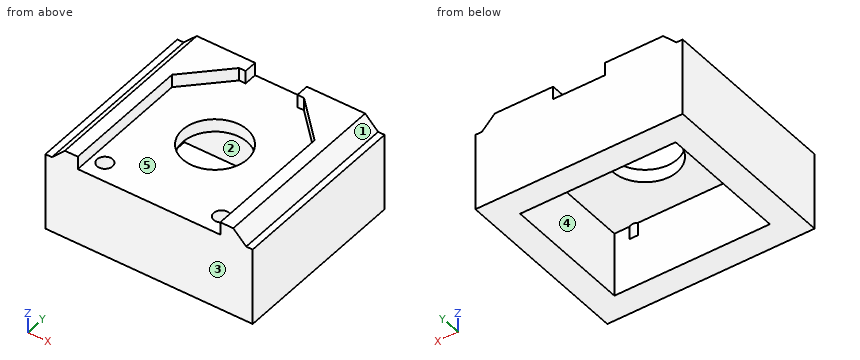
Autodesk Inventor part; units mm, degrees
ref_plane "YZ Plane" through (0, 0, 0) normal (1, 0, 0) x (0, 1, 0)
ref_plane "XZ Plane" through (0, 0, 0) normal (0, 1, 0) x (-1, 0, 0)
ref_plane "XY Plane" through (0, 0, 0) normal (0, 0, 1) x (1, 0, 0)
sketch "Sketch1" plane through (0, 0, 0) normal (0, 0, 1) x (1, 0, 0)
  line L0 (-14.0621, 11.3836) -> (-2.0621, 11.3836)
  line L1 (-2.0621, 11.3836) -> (-2.0621, 1.3836)
  line L2 (-2.0621, 1.3836) -> (-14.0621, 1.3836)
  line L3 (-14.0621, 1.3836) -> (-14.0621, 11.3836)
  line L4 (-0.0621, 13.3836) -> (-16.0621, 13.3836)
  line L5 (-16.0621, 13.3836) -> (-16.0621, -0.6164)
  line L6 (-16.0621, -0.6164) -> (-0.0621, -0.6164)
  line L7 (-0.0621, -0.6164) -> (-0.0621, 13.3836)
  point P0 (0, 0)
  dimension "d0" = 12
  dimension "d1" = 10
  dimension "d2" = 2
extrude "Extrusion1" add sketch "Sketch1" against normal blind 5
sketch "Sketch2" plane through (0, 0, 0) normal (0, 0, 1) x (1, 0, 0)
  line L0 (-0.0621, 13.3836) -> (-16.0621, 13.3836)
  line L1 (-0.0621, -0.6164) -> (-0.0621, 13.3836)
  line L2 (-16.0621, 13.3836) -> (-0.0621, 13.3836)
  line L3 (-0.0621, 13.3836) -> (-0.0621, -0.6164)
  line L4 (-0.0621, -0.6164) -> (-16.0621, -0.6164)
  line L5 (-16.0621, -0.6164) -> (-16.0621, 13.3836)
  line L6 (-0.0621, 13.3836) -> (-0.0621, -0.6164)
  line L7 (-0.0621, 6.3836) -> (-16.0621, 6.3836)
  line L8 (-16.0621, -0.6164) -> (-16.0621, 13.3836)
  circle A0 centre (-8.0621, 6.3836) radius 2.5
  point P0 (0, 0)
  dimension "d7" = 5
extrude "Extrusion2" add sketch "Sketch2" along normal blind 1 contours L1 L7 A0 L5 L0 | L1 L4 L5 L7 A0
sketch "Sketch3" plane through (0, 0, 1) normal (0, 0, 1) x (1, 0, 0)
  line L0 (-13.5621, 12.3836) -> (-2.5621, 12.3836)
  line L1 (-2.5621, 12.3836) -> (-2.5621, 0.3836)
  line L2 (-2.5621, 0.3836) -> (-13.5621, 0.3836)
  line L3 (-13.5621, 0.3836) -> (-13.5621, 12.3836)
  line L4 (-8.0621, 12.3836) -> (-8.0621, 0.3836)
  circle A0 centre (-8.0621, 6.3836) radius 2.5
  line L5 (-1.5621, 13.3836) -> (-14.5621, 13.3836)
  line L6 (-14.5621, 13.3836) -> (-14.5621, -0.6164)
  line L7 (-14.5621, -0.6164) -> (-1.5621, -0.6164)
  line L8 (-1.5621, -0.6164) -> (-1.5621, 13.3836)
  line L9 (-8.0621, 12.3836) -> (-10.0621, 12.3836)
  line L10 (-10.0621, 12.3836) -> (-10.0621, 13.3836)
  line L11 (-16.0621, 13.3836) -> (-0.0621, 13.3836)
  line L12 (-8.0621, 12.3836) -> (-6.0621, 12.3836)
  line L13 (-6.0621, 12.3836) -> (-6.0621, 13.3836)
  line L14 (-8.0621, 0.3836) -> (-4.0621, 0.3836)
  line L15 (-4.0621, 0.3836) -> (-4.0621, -0.6164)
  line L16 (-0.0621, -0.6164) -> (-16.0621, -0.6164)
  line L17 (-8.0621, 0.3836) -> (-12.0621, 0.3836)
  line L18 (-12.0621, 0.3836) -> (-12.0621, -0.6164)
  line L19 (-13.5621, 0.3836) -> (-13.5621, -0.6164)
  line L20 (-2.5621, 0.3836) -> (-2.5621, -0.6164)
  point P0 (0, 0)
  dimension "d8" = 11
  dimension "d9" = 12
  dimension "d10" = 1
  dimension "d11" = 2
  dimension "d12" = 2
  dimension "d13" = 4
  dimension "d14" = 4
extrude "Extrusion3" add sketch "Sketch3" along normal blind 1 contours L3 L19 L7 L6 L5 L10 L0 | L13 L5 L8 L7 L20 L1 L0
chamfer "Chamfer1" distance 1 angle 45 2 edges at (-14.5621, 6.3836, 1) (-1.5621, 6.3836, 1)
chamfer "Chamfer2" distance 3 angle 45 2 edges at (-13.5621, 12.3836, 1.5) (-2.5621, 12.3836, 1.5)
sketch "Sketch4" plane through (0, 0, 1) normal (0, 0, 1) x (1, 0, 0)
  circle A0 centre (-12.5621, 0.8836) radius 0.6
  circle A1 centre (-3.5621, 0.8836) radius 0.6
  line L0 (-12.5621, 0.8836) -> (-3.5621, 0.8836)
  circle A2 centre (-8.0621, 6.3836) radius 2.5
  line L1 (-8.0621, 0.8836) -> (-8.0621, 6.3836)
  point P0 (0, 0)
  dimension "d23" = 1.2
  dimension "d24" = 1.2
  dimension "d25" = 5.5
  dimension "d26" = 9
extrude "Extrusion4" cut sketch "Sketch4" against normal blind 2 contours A0 | A1
properties part number "pid_test_structure"
CAD build for the part. Positions are in the model's coordinates, mm. Face numbers are marked on the shaded views. A direction names the side the tool comes from. Coordinates: 2 decimals unless noted, no trailing zeros. Order: outer loops, then holes, each group sorted by start corner. A loop starts at its lowest first (then second) coordinate and runs counter-clockwise, first axis right, second up. Notation, with made-up numbers: (25, 0) -> (82, 0) arc R15 cw to (82, 15) -> close; hole circle Ø1 at (-27, -29.75). An arc over 180 degrees is marked (long way). Answer in a Markdown table with one row per item.
1) Band-saw the part on C-C (z = 1.25). List the corners of the cut face in (x, y).
Check values:
| item | result |
|---|---|
| outline | (-15.31, -0.62) -> (-13.56, -0.62) -> (-13.56, 9.38) -> (-10.56, 12.38) -> (-10.06, 12.38) -> (-10.06, 13.38) -> (-15.31, 13.38) -> close; (-6.06, 12.38) -> (-5.56, 12.38) -> (-2.56, 9.38) -> (-2.56, -0.62) -> (-0.81, -0.62) -> (-0.81, 13.38) -> (-6.06, 13.38) -> close |
2) Drill centre lines: line 1 (X direction, y = 4.5, z = -2.5); line 2 (Y direction, x = -9, z = -4.25); line 3 (Z direction, x = -2.25, y = 9). Where is each one in solid material? Low to high.
Check values:
| item | result |
|---|---|
| line 1 | -16.06 to -14.06, -2.06 to -0.06 |
| line 2 | -0.62 to 1.38, 11.38 to 13.38 |
| line 3 | 0 to 2 |
3) Flat gauge pins, fed straight in: P1, Ø0.6, axis at x = -3.5, y = 0.5, coming from the +Z side; P2, Ø0.5, axis at y = 2, z = 1.5, coming from the -X side; P3, Ø0.5, axis at y = 13, z = 1.5, coming from the +X side; P4, Ø4.5, axis at x = -8.06, y = 6.38, coming from the +Z side. Where does each tip first touch, or does it go through?
Check values:
| item | result |
|---|---|
| P1 | z = 1 |
| P2 | x = -15.31 |
| P3 | x = -0.81 |
| P4 | through |
4) Band-saw the part on B-B (z = -3). List the corners of the cut face in (x, y), and give its area (3 significant figures).
Check values:
| item | result |
|---|---|
| outline | (-16.06, -0.62) -> (-0.06, -0.62) -> (-0.06, 13.38) -> (-16.06, 13.38) -> close; hole (-14.06, 1.38) -> (-2.06, 1.38) -> (-2.06, 11.38) -> (-14.06, 11.38) -> close |
| area | 104 mm2 |
5) Which spindle directions (+Z, -Z, +X, -X, +Y, -Y) get a long thin tool onto all of the face, cutting with end or side? Do the marked faces 1 and 2. Say none if no direction does.
Check values:
| item | result |
|---|---|
| face 1 | +Z, +X, +Y, -Y |
| face 2 | -Z |
6) Band-saw the part on D-D (x = -6.5). List the corners of the cut face in (y, z), and give its area (3 significant figures).
Check values:
| item | result |
|---|---|
| outline | (-0.62, -5) -> (1.38, -5) -> (1.38, 0) -> (4.43, 0) -> (4.43, 1) -> (-0.62, 1) -> close; (8.34, 0) -> (11.38, 0) -> (11.38, -5) -> (13.38, -5) -> (13.38, 1) -> (8.34, 1) -> close |
| area | 30.1 mm2 |
7) Mould opens along Y. For the marked faces 3, 4 and 5 say: pulls with the +Y half, pulls with the -Y half, needs draft (parallel to the pull), parting line crosses it, or undercut.
Check values:
| item | result |
|---|---|
| face 3 | pulls with the -Y half |
| face 4 | undercut |
| face 5 | needs draft |
